Geometry: final body of the model. Coordinates: model frame, mm. Face numbers are marked on the shaded views. A direction names the side the tool comes from. Give positions to 0.01 mm unless a question says otherwise; leave off trailing zeros. Write each loop counter-clockwise with the first axis right and the second up, starting at its lowest first coordinate (ties: lowest second). Pieces come first, ordered by that corner, then holes.
Q1. Cut plane B-B on x = 2. Return the cut outline in (y, z), plus the area to 3 significant figures.
Q2. Cut plane D-D on z = 2.5. Return the cut outline in (x, y).
Q3. Line query: L1, parallel to Z at x = 0.25, y = -6; L2, parallel to X at y = 0.5, z = 3; L3, parallel to X at y = -0.75, z = 4.5. Output: solid intervals per line, ascending.
Q4. Reachability of the marked faces 1 and 2 from +Z, -Z, +X, -X, +Y, -Y: full face, straight path, thin tool, end or side. Return the list, or none.
Q5. Cut plane C-C on y = 0.5. Return the cut outline in (x, z), plus the area to 3 significant figures.
Q6. Pin query (flat end, axial travel): pin 1 (4 mm diameter, centred on x = 4.5, z = 4, fed in from +Y); pin 2 (1 mm diameter, centred on y = -1.5, z = 1.5, fed in from -X); pin 3 (3 mm diameter, centred on x = 0, z = 7, fed in from -Y); pin 4 (4 mm diameter, centred on x = 0.5, y = 2.5, fed in from +Z). Return the tip coordinate at first contact, or that it passes through.
Q7. Cut plane A-A on z = 7. Return the cut outline in (x, y).
```python
from build123d import *

# Parameters (mm, degrees)
F1_DEPTH = 1.397
F2_DEPTH = 8.7376
F3_DEPTH = 4.2926


# Not quite as in the source:
# - ends of sketch curves that miss each other by under 0.0002 mm in the source are joined


with BuildPart() as f1:
    # F0 (on Top) → F1 (new body)
    with BuildSketch(Plane.XY):
        with BuildLine():
            ThreePointArc((-5.4345187307, 0), (-3.8427850469, 3.8427850469), (0, 5.4345187307))
            Line((0, 5.4345187307), (0, 6.7959154799))
            ThreePointArc((0, 6.7959154799), (-2.5520653679, 6.2985259837), (-4.7305620794, 4.8791648489))
            ThreePointArc((-4.7305620794, 4.8791648489), (-7.3841557332, 3.3252325154), (-10.4555039298, 3.1733212198))
            ThreePointArc((-10.4555039298, 3.1733212198), (-10.7604870325, 3.2172453575), (-11.0682662539, 3.2319337461))
            Line((-11.0682662539, 3.2319337461), (-11.0682662539, 1.438874613))
            ThreePointArc((-11.0682662539, 1.438874613), (-10.0508282577, 1.0174379961), (-9.6293916409, 0))
            Line((-9.6293916409, 0), (-5.4345187307, 0))
        make_face()
        with BuildLine():
            ThreePointArc((-12.5071408669, 0), (-12.08570425, 1.0174379961), (-11.0682662539, 1.438874613))
            Line((-11.0682662539, 1.438874613), (-11.0682662539, 3.2319337461))
            ThreePointArc((-11.0682662539, 3.2319337461), (-13.3535885221, 2.2853222682), (-14.3002, 0))
            Line((-14.3002, 0), (-12.5071408669, 0))
        make_face()
        with BuildLine():
            Line((-11.0682662539, -3.2319337461), (-11.0682662539, -1.438874613))
            ThreePointArc((-11.0682662539, -1.438874613), (-12.08570425, -1.0174379961), (-12.5071408669, 0))
            Line((-12.5071408669, 0), (-14.3002, 0))
            ThreePointArc((-14.3002, 0), (-13.3535885221, -2.2853222682), (-11.0682662539, -3.2319337461))
        make_face()
        with BuildLine():
            Line((0, -6.7959154799), (0, -5.4345187307))
            ThreePointArc((0, -5.4345187307), (-3.8427850469, -3.8427850469), (-5.4345187307, 0))
            Line((-5.4345187307, 0), (-9.6293916409, 0))
            ThreePointArc((-9.6293916409, 0), (-10.0508282577, -1.0174379961), (-11.0682662539, -1.438874613))
            Line((-11.0682662539, -1.438874613), (-11.0682662539, -3.2319337461))
            ThreePointArc((-11.0682662539, -3.2319337461), (-10.7604870325, -3.2172453575), (-10.4555053814, -3.1733137022))
            ThreePointArc((-10.4555053814, -3.1733137022), (-7.3841557332, -3.3252325154), (-4.7305659764, -4.8791688684))
            ThreePointArc((-4.7305659764, -4.8791688684), (-2.5520653679, -6.2985259837), (0, -6.7959154799))
        make_face()
        with BuildLine():
            ThreePointArc((0, -5.4345187307), (3.8427850469, -3.8427850469), (5.4345187307, 0))
            Line((5.4345187307, 0), (4.5601256966, 0))
            ThreePointArc((4.5601256966, 0), (3.2244958031, -3.2244958031), (0, -4.5601256966))
            Line((0, -4.5601256966), (0, -5.4345187307))
        make_face()
        with BuildLine():
            ThreePointArc((-5.4345187307, 0), (-3.8427850469, -3.8427850469), (0, -5.4345187307))
            Line((0, -5.4345187307), (0, -4.5601256966))
            ThreePointArc((0, -4.5601256966), (-3.2244958031, -3.2244958031), (-4.5601256966, 0))
            Line((-4.5601256966, 0), (-5.4345187307, 0))
        make_face()
        with BuildLine():
            Line((0, 4.5601256966), (0, 5.4345187307))
            ThreePointArc((0, 5.4345187307), (-3.8427850469, 3.8427850469), (-5.4345187307, 0))
            Line((-5.4345187307, 0), (-4.5601256966, 0))
            ThreePointArc((-4.5601256966, 0), (-3.2244958031, 3.2244958031), (0, 4.5601256966))
        make_face()
        with BuildLine():
            Line((4.5601256966, 0), (5.4345187307, 0))
            ThreePointArc((5.4345187307, 0), (3.8427850469, 3.8427850469), (0, 5.4345187307))
            Line((0, 5.4345187307), (0, 4.5601256966))
            ThreePointArc((0, 4.5601256966), (3.2244958031, 3.2244958031), (4.5601256966, 0))
        make_face()
        with BuildLine():
            ThreePointArc((0, 5.4345187307), (3.8427850469, 3.8427850469), (5.4345187307, 0))
            Line((5.4345187307, 0), (9.6293916409, 0))
            ThreePointArc((9.6293916409, 0), (10.0508282577, 1.0174379961), (11.0682662539, 1.438874613))
            Line((11.0682662539, 1.438874613), (11.0682662539, 3.2319337461))
            ThreePointArc((11.0682662539, 3.2319337461), (10.7604870325, 3.2172453575), (10.4555053814, 3.1733137022))
            ThreePointArc((10.4555053814, 3.1733137022), (7.3841557332, 3.3252325154), (4.7305659764, 4.8791688684))
            ThreePointArc((4.7305659764, 4.8791688684), (2.5520653679, 6.2985259837), (0, 6.7959154799))
            Line((0, 6.7959154799), (0, 5.4345187307))
        make_face()
        with BuildLine():
            Line((9.6293916409, 0), (5.4345187307, 0))
            ThreePointArc((5.4345187307, 0), (3.8427850469, -3.8427850469), (0, -5.4345187307))
            Line((0, -5.4345187307), (0, -6.7959154799))
            ThreePointArc((0, -6.7959154799), (2.5520653679, -6.2985259837), (4.7305620794, -4.8791648489))
            ThreePointArc((4.7305620794, -4.8791648489), (7.3841557332, -3.3252325154), (10.4555039298, -3.1733212198))
            ThreePointArc((10.4555039298, -3.1733212198), (10.7604870325, -3.2172453575), (11.0682662539, -3.2319337461))
            Line((11.0682662539, -3.2319337461), (11.0682662539, -1.438874613))
            ThreePointArc((11.0682662539, -1.438874613), (10.0508282577, -1.0174379961), (9.6293916409, 0))
        make_face()
        with BuildLine():
            ThreePointArc((12.5071408669, 0), (12.08570425, -1.0174379961), (11.0682662539, -1.438874613))
            Line((11.0682662539, -1.438874613), (11.0682662539, -3.2319337461))
            ThreePointArc((11.0682662539, -3.2319337461), (13.3535885221, -2.2853222682), (14.3002, 0))
            Line((14.3002, 0), (12.5071408669, 0))
        make_face()
        with BuildLine():
            Line((11.0682662539, 3.2319337461), (11.0682662539, 1.438874613))
            ThreePointArc((11.0682662539, 1.438874613), (12.08570425, 1.0174379961), (12.5071408669, 0))
            Line((12.5071408669, 0), (14.3002, 0))
            ThreePointArc((14.3002, 0), (13.3535885221, 2.2853222682), (11.0682662539, 3.2319337461))
        make_face()
    extrude(amount=F1_DEPTH)

    # F0 (on Top) → F2 (join)
    with BuildSketch(Plane.XY):
        with BuildLine():
            Line((0, 3.6514210372), (0, 4.5601256966))
            ThreePointArc((0, 4.5601256966), (-3.2244958031, 3.2244958031), (-4.5601256966, 0))
            Line((-4.5601256966, 0), (-3.6514210372, 0))
            ThreePointArc((-3.6514210372, 0), (-2.5819445763, 2.5819445763), (0, 3.6514210372))
        make_face()
        with BuildLine():
            Line((3.6514210372, 0), (4.5601256966, 0))
            ThreePointArc((4.5601256966, 0), (3.2244958031, 3.2244958031), (0, 4.5601256966))
            Line((0, 4.5601256966), (0, 3.6514210372))
            ThreePointArc((0, 3.6514210372), (2.5819445763, 2.5819445763), (3.6514210372, 0))
        make_face()
        with BuildLine():
            ThreePointArc((0, -4.5601256966), (3.2244958031, -3.2244958031), (4.5601256966, 0))
            Line((4.5601256966, 0), (3.6514210372, 0))
            ThreePointArc((3.6514210372, 0), (2.5819445763, -2.5819445763), (0, -3.6514210372))
            Line((0, -3.6514210372), (0, -4.5601256966))
        make_face()
        with BuildLine():
            ThreePointArc((-4.5601256966, 0), (-3.2244958031, -3.2244958031), (0, -4.5601256966))
            Line((0, -4.5601256966), (0, -3.6514210372))
            ThreePointArc((0, -3.6514210372), (-2.5819445763, -2.5819445763), (-3.6514210372, 0))
            Line((-3.6514210372, 0), (-4.5601256966, 0))
        make_face()
    extrude(amount=F2_DEPTH)

    # F0 (on Top) → F3 (join)
    with BuildSketch(Plane.XY):
        with BuildLine():
            ThreePointArc((-5.4345187307, 0), (-3.8427850469, -3.8427850469), (0, -5.4345187307))
            Line((0, -5.4345187307), (0, -4.5601256966))
            ThreePointArc((0, -4.5601256966), (-3.2244958031, -3.2244958031), (-4.5601256966, 0))
            Line((-4.5601256966, 0), (-5.4345187307, 0))
        make_face()
        with BuildLine():
            ThreePointArc((0, -5.4345187307), (3.8427850469, -3.8427850469), (5.4345187307, 0))
            Line((5.4345187307, 0), (4.5601256966, 0))
            ThreePointArc((4.5601256966, 0), (3.2244958031, -3.2244958031), (0, -4.5601256966))
            Line((0, -4.5601256966), (0, -5.4345187307))
        make_face()
        with BuildLine():
            Line((4.5601256966, 0), (5.4345187307, 0))
            ThreePointArc((5.4345187307, 0), (3.8427850469, 3.8427850469), (0, 5.4345187307))
            Line((0, 5.4345187307), (0, 4.5601256966))
            ThreePointArc((0, 4.5601256966), (3.2244958031, 3.2244958031), (4.5601256966, 0))
        make_face()
        with BuildLine():
            Line((0, 4.5601256966), (0, 5.4345187307))
            ThreePointArc((0, 5.4345187307), (-3.8427850469, 3.8427850469), (-5.4345187307, 0))
            Line((-5.4345187307, 0), (-4.5601256966, 0))
            ThreePointArc((-4.5601256966, 0), (-3.2244958031, 3.2244958031), (0, 4.5601256966))
        make_face()
    extrude(amount=F3_DEPTH)


solid = f1.part
```
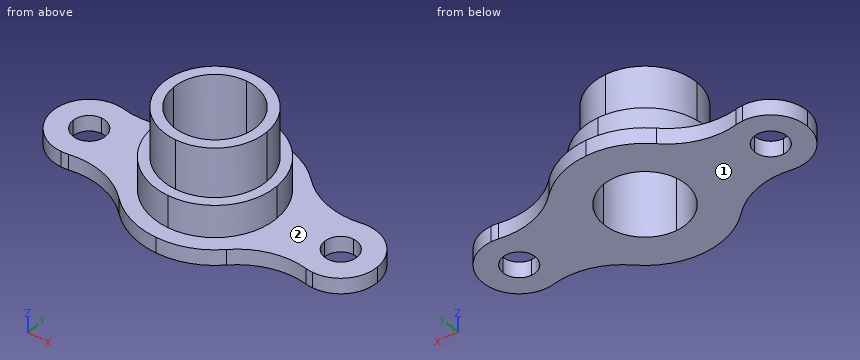
Data:
1. outline: (-6.49, 0) - (-3.05, 0) - (-3.05, 8.74) - (-4.1, 8.74) - (-4.1, 4.29) - (-5.05, 4.29) - (-5.05, 1.4) - (-6.49, 1.4) - close; (3.05, 0) - (6.49, 0) - (6.49, 1.4) - (5.05, 1.4) - (5.05, 4.29) - (4.1, 4.29) - (4.1, 8.74) - (3.05, 8.74) - close
1. area: 30.5 mm2
2. outline: circle Ø10.87 at (0, 0); hole circle Ø7.3 at (0, 0)
3. L1: z = 0 to 1.4
3. L2: x = -5.41 to -3.62, 3.62 to 5.41
3. L3: x = -4.5 to -3.57, 3.57 to 4.5
4. face 1: -Z, +X, -X, +Y, -Y
4. face 2: +Z
5. outline: (-14.26, 0) - (-12.42, 0) - (-12.42, 1.4) - (-14.26, 1.4) - close; (-9.72, 0) - (-3.62, 0) - (-3.62, 8.74) - (-4.53, 8.74) - (-4.53, 4.29) - (-5.41, 4.29) - (-5.41, 1.4) - (-9.72, 1.4) - close; (3.62, 0) - (9.72, 0) - (9.72, 1.4) - (5.41, 1.4) - (5.41, 4.29) - (4.53, 4.29) - (4.53, 8.74) - (3.62, 8.74) - close; (12.42, 0) - (14.26, 0) - (14.26, 1.4) - (12.42, 1.4) - close
5. area: 40.7 mm2
6. pin 1: stops at y = 4.83
6. pin 2: stops at x = -14.14
6. pin 3: stops at y = -4.56
6. pin 4: stops at z = 8.74
7. outline: circle Ø9.12 at (0, 0); hole circle Ø7.3 at (0, 0)
